from build123d import *

# Parameters (mm, degrees)
SKETCH_1_W                = 15
SKETCH_1_H                = 15
SKETCH_1_W_2              = 12
SKETCH_1_H_2              = 12
EXTRUDE_1_DEPTH           = 200
CUT_EXTRUDE_START         = -7.5
CUT_EXTRUDE_1_OUTLINE_R   = 1.5
CUT_EXTRUDE_1_OUTLINE_R_2 = 2
CUT_EXTRUDE_1_DEPTH       = 15


# Read off the part's stored shape, not the designer's step: 切除-拉伸1
with BuildPart() as part:
    # 草图1 → 凸台-拉伸1 (new body)
    with BuildSketch(Plane(origin=(0, 0, 0), x_dir=(1, 0, 0), z_dir=(0, 1, 0))):
        Rectangle(SKETCH_1_W, SKETCH_1_H)
        Rectangle(SKETCH_1_W_2, SKETCH_1_H_2, mode=Mode.SUBTRACT)
    extrude(amount=EXTRUDE_1_DEPTH)

    # 切除-拉伸1 outline → 切除-拉伸1 (cut)
    with BuildSketch(Plane.YZ.offset(CUT_EXTRUDE_START)):
        with Locations((12.5, 0)):
            Circle(CUT_EXTRUDE_1_OUTLINE_R)
        with Locations((32.5, 0)):
            Circle(CUT_EXTRUDE_1_OUTLINE_R)
        with Locations((52.5, 0)):
            Circle(CUT_EXTRUDE_1_OUTLINE_R_2)
        with Locations((147.5, 0)):
            Circle(CUT_EXTRUDE_1_OUTLINE_R_2)
        with Locations((167.5, 0)):
            Circle(CUT_EXTRUDE_1_OUTLINE_R)
        with Locations((187.5, 0)):
            Circle(CUT_EXTRUDE_1_OUTLINE_R)
    extrude(amount=CUT_EXTRUDE_1_DEPTH, mode=Mode.SUBTRACT)


solid = part.part
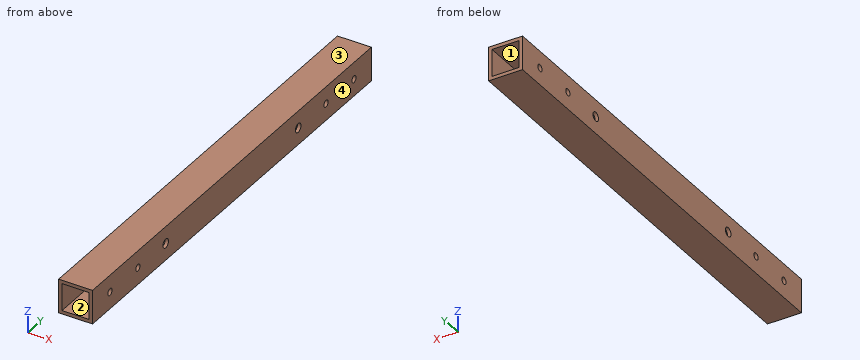
CAD build for the part. Positions are in the model's coordinates, mm. Face numbers are marked on the shaded views. Coordinates: 2 decimals unless noted, no trailing zeros. Write each loop counter-clockwise with the first axis right and the second up, starting at its lowest first coordinate (ties: lowest second). Pieces come first, ordered by that corner, then holes. Notation, with made-up numbers: M -2.75,53.5 L 26.25,53.5 A31 ccw 26.25,82.5 Z; hole C -1.75,-13.75 d2. An arc over 180 degrees is marked long. Answer as a JSON object with one key per item and string values. Group by question number.
1) Pin check, flat tip, straight feed: pin 1 Ø2.5 at (y, z) = (167.5, 0) entering from +X. Stop position of the tip, or through.
2) Saw through at A-A (y = 52.5). Write the cut outline in (x, z), plus the area to 3 significant figures.
3) Saw through at C-C (y = 28). Write the cut outline in (x, z).
4) Saw through at B-B (x = 1.75). Write the cut outline in (y, z).
5) Mould opens along X. For the marked faces 1, 2, 3 and 4 say: +X half, -X half, draft (parallel to the pull), parting line (faces both ways), or undercut.
6) Wall check: line 1 (Z direction, x = 6.35, y = 52.5); line 2 (X direction, y = 86.5, z = 4); line 3 (Z direction, x = -6.65, y = 12.5). Give the ranges that are in metal, low to high. Write a range as from..to.
Values follow:
{
 "1": {"pin 1": "passes through"},
 "2": {"outline": "M -7.5,-7.5 L 7.5,-7.5 L 7.5,-2 L 6,-2 L 6,-6 L -6,-6 L -6,-2 L -7.5,-2 Z; M -7.5,2 L -6,2 L -6,6 L 6,6 L 6,2 L 7.5,2 L 7.5,7.5 L -7.5,7.5 Z", "area": "69.0 mm2"},
 "3": {"outline": "M -7.5,-7.5 L 7.5,-7.5 L 7.5,7.5 L -7.5,7.5 Z; hole M -6,-6 L 6,-6 L 6,6 L -6,6 Z"},
 "4": {"outline": "M 0,-7.5 L 200,-7.5 L 200,-6 L 0,-6 Z; M 0,6 L 200,6 L 200,7.5 L 0,7.5 Z"},
 "5": {"face 1": "undercut", "face 2": "undercut", "face 3": "draft", "face 4": "+X half"},
 "6": {"line 1": "z = -7.5..-2, 2..7.5", "line 2": "x = -7.5..-6, 6..7.5", "line 3": "z = -7.5..-1.5, 1.5..7.5"}
}
